Geometry: final body of the model. Coordinates: model frame, mm. Give positions to 0.01 mm unless a question says otherwise; leave off trailing zeros. Loops run counter-clockwise (first coordinate to the right, second up) from the corner with the lowest first, then second, coordinate; pieces in that order, holes last.
1. Material intervals for line 1 along Y through (x, z) = (-42, 2); line 2 along Y through (x, z) = (45, 1); line 3 along X through (y, z) = (-3, 4.25), sorted ascending.
2. Section A-A, the plane x = -56.5. Output: boundary loops of the cut face in (y, z), then the cut area to 3 significant figures.
3. Section C-C, the plane z = 1.5. Output: boundary loops of the cut face in (x, y).
4. Section B-B, the plane y = 1. Output: boundary loops of the cut face in (x, z).
from build123d import *

# Parameters (mm, degrees)
F1_DEPTH = 6.35
F3_DEPTH = 6.351
F5_DEPTH = 6.351


with BuildPart() as f1:
    # F0 (on Top) → F1 (new body)
    with BuildSketch(Plane.XY):
        with BuildLine():
            Line((113.9825, 84.1375), (-113.9825, 84.1375))
            ThreePointArc((-113.9825, 84.1375), (-117.574602, 82.649602), (-119.0625, 79.0575))
            Line((-119.0625, 79.0575), (-119.0625, -79.0575))
            ThreePointArc((-119.0625, -79.0575), (-117.574602, -82.649602), (-113.9825, -84.1375))
            Line((-113.9825, -84.1375), (113.9825, -84.1375))
            ThreePointArc((113.9825, -84.1375), (117.574602, -82.649602), (119.0625, -79.0575))
            Line((119.0625, -79.0575), (119.0625, 79.0575))
            ThreePointArc((119.0625, 79.0575), (117.574602, 82.649602), (113.9825, 84.1375))
        make_face()
    extrude(amount=F1_DEPTH)

    # F2 (on face) → F3 (cut, through all)
    with BuildSketch(Plane.XY.offset(6.35)):
        Polygon((0, 46.305061), (-89.802561, -43.4975), (89.802561, -43.4975), align=None)
    extrude(amount=-F3_DEPTH, mode=Mode.SUBTRACT)

    # F4 (on face) → F5 (cut, through all)
    with BuildSketch(Plane.XY.offset(6.35)):
        with BuildLine():
            ThreePointArc((0.556776, 47.544337), (0, 47.774961), (-0.556776, 47.544337))
            Line((-0.556776, 47.544337), (-91.524437, -43.423324))
            ThreePointArc((-91.524437, -43.423324), (-91.695123, -44.281425), (-90.967661, -44.7675))
            Line((-90.967661, -44.7675), (90.967661, -44.7675))
            ThreePointArc((90.967661, -44.7675), (91.695123, -44.281425), (91.524437, -43.423324))
            Line((91.524437, -43.423324), (0.556776, 47.544337))
        make_face()
    extrude(amount=-F5_DEPTH, mode=Mode.SUBTRACT)


solid = f1.part
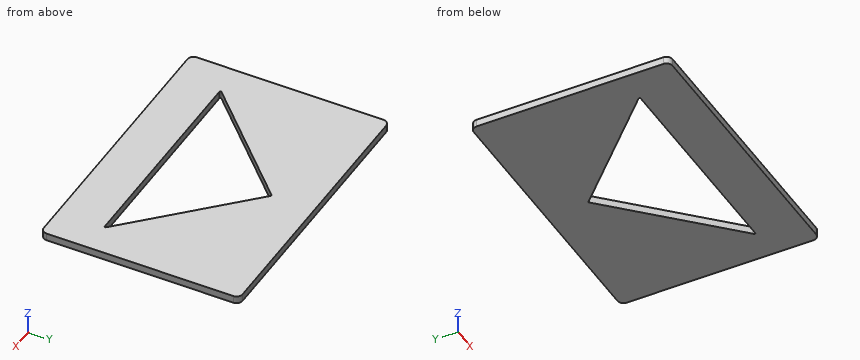
Answers below:
1. line 1: y = -84.14 to -44.77, 6.1 to 84.14
1. line 2: y = -84.14 to -44.77, 3.1 to 84.14
1. line 3: x = -119.06 to -51.1, 51.1 to 119.06
2. outline: (-84.14, 0) - (-44.77, 0) - (-44.77, 6.35) - (-84.14, 6.35) - close; (-8.4, 0) - (84.14, 0) - (84.14, 6.35) - (-8.4, 6.35) - close
2. area: 838 mm2
3. outline: (-119.06, -79.06) arc R5.08 ccw to (-113.98, -84.14) - (113.98, -84.14) arc R5.08 ccw to (119.06, -79.06) - (119.06, 79.06) arc R5.08 ccw to (113.98, 84.14) - (-113.98, 84.14) arc R5.08 ccw to (-119.06, 79.06) - close; hole (-91.52, -43.42) arc R0.79 ccw to (-90.97, -44.77) - (90.97, -44.77) arc R0.79 ccw to (91.52, -43.42) - (0.56, 47.54) arc R0.79 ccw to (-0.56, 47.54) - close
4. outline: (-119.06, 0) - (-47.1, 0) - (-47.1, 6.35) - (-119.06, 6.35) - close; (47.1, 0) - (119.06, 0) - (119.06, 6.35) - (47.1, 6.35) - close
